Could you check a few things on this model? Use its own coordinates, in mm. A direction names the side the tool comes from. Give positions to 0.01 mm unless a question says otherwise; leave off trailing zeros. Loops run counter-clockwise (first coordinate to the right, second up) from the corner with the lowest first, then second, coordinate; pieces in that order, holes last. Notation, with made-up numbers: (5, -26.75) - (61, -26.75) arc R27 ccw to (61, -7.75) - close; hole circle Ø9 at (-38, 51.5). An arc over 180 degrees is marked (long way). Use CSV: the item, a comma, the result in double quotes.
from build123d import *

# Parameters (mm, degrees)
SKETCH_W        = 105
SKETCH_H        = 60.5
PAD_DEPTH       = 2
SKETCH001_W     = 100
SKETCH001_H     = 55.5
PAD001_DEPTH    = 1
SKETCH002_R     = 3.5
POCKET_DEPTH    = 1
SKETCH003_R     = 1.75
POCKET001_DEPTH = 3.001


with BuildPart() as part:
    # Sketch → Pad (new body)
    with BuildSketch(Plane.XY):
        with Locations((52.5, 30.25)):
            Rectangle(SKETCH_W, SKETCH_H)
    extrude(amount=PAD_DEPTH)

    # Sketch001 → Pad001 (new body)
    with BuildSketch(Plane(origin=(0, 0, 0), x_dir=(1, 0, 0), z_dir=(0, 0, -1))):
        with Locations((52.5, -30.25)):
            Rectangle(SKETCH001_W, SKETCH001_H)
    extrude(amount=PAD001_DEPTH)

    # Sketch002 → Pocket (cut)
    with BuildSketch(Plane(origin=(0, 0, -1), x_dir=(1, 0, 0), z_dir=(0, 0, -1))):
        with Locations((3.5, -3.5)):
            Circle(SKETCH002_R)
        with Locations((3.5, -57)):
            Circle(SKETCH002_R)
        with Locations((101.5, -3.5)):
            Circle(SKETCH002_R)
        with Locations((101.5, -57)):
            Circle(SKETCH002_R)
    extrude(amount=-POCKET_DEPTH, mode=Mode.SUBTRACT)

    # Sketch003 → Pocket001 (cut, through all)
    with BuildSketch(Plane.XY.offset(2)):
        with Locations((3.5, 57)):
            Circle(SKETCH003_R)
        with Locations((101.5, 57)):
            Circle(SKETCH003_R)
        with Locations((3.5, 3.5)):
            Circle(SKETCH003_R)
        with Locations((101.5, 3.5)):
            Circle(SKETCH003_R)
    extrude(amount=-POCKET001_DEPTH, mode=Mode.SUBTRACT)


solid = part.part
1) I need wall thicknesses on line 1 along Y through (x, z) = (101.5, 1.1); line 2 along Y through (x, z) = (58, -0.2); line 3 along X through (y, z) = (24.5, -0.7). Which ranges of each line are inside material? Lowest first, please.
Answer below:
line 1,"y = 0 to 1.75, 5.25 to 55.25, 58.75 to 60.5"
line 2,"y = 2.5 to 58"
line 3,"x = 2.5 to 102.5"
2) Suppose I cut it at D-D (x = 55). Please give me the cut outline in (y, z).
Answer below:
outline,"(0, 0) - (2.5, 0) - (2.5, -1) - (58, -1) - (58, 0) - (60.5, 0) - (60.5, 2) - (0, 2) - close"
3) We'd pull the mould along Y, two halves only. Please class faces 3 (the cylindrical face through (98.99, 5.94, -0.51)), 4 (the flat face through (52, 0, 1)), 5 (the flat face through (52, 60.5, 1)): +Y half, -Y half, draft (parallel to the pull), parting line (faces both ways), or undercut.
Answer below:
face 3,"undercut"
face 4,"-Y half"
face 5,"+Y half"
4) I'm going to push flat-ended pins straight in: P1, Ø5.5, axis at x = 3.5, y = 3.5, coming from the -Z side; P2, Ø0.8, axis at x = 65, z = -0.5, coming from the -Y side; P3, Ø0.5, axis at y = 40.5, z = -0.5, coming from the -X side. Where does each tip first touch, or does it pass through?
Answer below:
P1,"stops at z = 0"
P2,"stops at y = 2.5"
P3,"stops at x = 2.5"
5) Suppose I cut it at A-A (x = 101.5). Please give me the cut outline in (y, z), plus the area to 4 significant figures.
Answer below:
outline,"(0, 0) - (1.75, 0) - (1.75, 2) - (0, 2) - close; (5.25, 0) - (7, 0) - (7, -1) - (53.5, -1) - (53.5, 0) - (55.25, 0) - (55.25, 2) - (5.25, 2) - close; (58.75, 0) - (60.5, 0) - (60.5, 2) - (58.75, 2) - close"
area,"153.5 mm2"
6) Suppose I cut it at B-B (y = 57). Please give me the cut outline in (x, z).
Answer below:
outline,"(0, 0) - (1.75, 0) - (1.75, 2) - (0, 2) - close; (5.25, 0) - (7, 0) - (7, -1) - (98, -1) - (98, 0) - (99.75, 0) - (99.75, 2) - (5.25, 2) - close; (103.25, 0) - (105, 0) - (105, 2) - (103.25, 2) - close"
7) Which directions (+Z, -Z, +X, -X, +Y, -Y) give clear straight access to the entire face, cutting with the end or side of a thin tool? Please do faces 1 (the cylindrical face through (6.01, 54.56, -0.51)), 2 (the cylindrical face through (2.11, 2.44, 1.01)).
Answer below:
face 1,"-Z"
face 2,"+Z, -Z"
8) Suppose I cut it at C-C (y = 23). Please give me the cut outline in (x, z).
Answer below:
outline,"(0, 0) - (2.5, 0) - (2.5, -1) - (102.5, -1) - (102.5, 0) - (105, 0) - (105, 2) - (0, 2) - close"
